Autodesk Inventor part; units mm, degrees
ref_plane "YZ Plane" through (0, 0, 0) normal (1, 0, 0) x (0, 1, 0)
ref_plane "XZ Plane" through (0, 0, 0) normal (0, 1, 0) x (-1, 0, 0)
ref_plane "XY Plane" through (0, 0, 0) normal (0, 0, 1) x (1, 0, 0)
sketch "Sketch1" plane through (0, 0, 0) normal (0, 0, 1) x (1, 0, 0)
  line L0 (0, 0) -> (30, 0)
  line L1 (30, 0) -> (30, 15)
  line L2 (30, 15) -> (0, 15)
  line L3 (0, 15) -> (0, 0)
  dimension "d0" = 30
  dimension "d1" = 15
extrude "Extrusion1" add sketch "Sketch1" along normal blind 25
sketch "Sketch2" plane through (0, 15, 0) normal (0, 1, 0) x (1, 0, 0)
  line L0 (30, 0) -> (0, 0)
  line L1 (0, 0) -> (0, -25)
  line L2 (30, -25) -> (0, -25)
  line L3 (30, 0) -> (30, -25)
  line L4 (7, -25) -> (23, -25)
  line L5 (23, -25) -> (23, -6)
  line L6 (23, -6) -> (7, -6)
  line L7 (7, -6) -> (7, -25)
  point P0 (0, 0)
  dimension "d5" = 16
  dimension "d27" = 7
  dimension "d28" = 6
extrude "Extrusion2" cut sketch "Sketch2" against normal up to next contours L2 L7 L6 L5
sketch "Sketch3" plane through (30, 0, 0) normal (1, 0, 0) x (0, 0, -1)
  circle A0 centre (-17.5, 7.5) radius 2.5
  line L0 (-25, 0) -> (-25, 15)
  line L1 (0, 15) -> (-25, 15)
  point P0 (0, 0)
  dimension "d10" = 5
  dimension "d11" = 7.5
  dimension "d12" = 7.5
extrude "Extrusion3" cut sketch "Sketch3" against normal through all
sketch "Sketch6" plane through (7, 15, 6) normal (0, 0, 1) x (1, 0, 0)
  circle A0 centre (8, -7.5) radius 5
  line L0 (0, 0) -> (16, 0)
  line L1 (16, 0) -> (16, -15)
  point P0 (-7, -15)
  dimension "d29" = 10
  dimension "d30" = 7.5
  dimension "d31" = 8
extrude "Extrusion6" cut sketch "Sketch6" against normal blind 4
sketch "Sketch7" plane through (15, 7.5, 2) normal (0, 0, 1) x (1, 0, 0)
  circle A0 centre (0, 0) radius 3.5
  point P0 (-15, -7.5)
  dimension "d34" = 7
extrude "Extrusion7" cut sketch "Sketch7" against normal up to next
properties part number "Arm_Pulley_Connector"
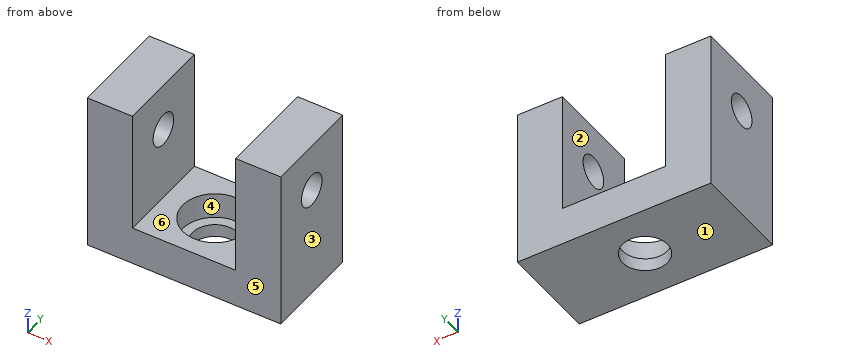
Geometry check sheet. Reference: the model listing, model coordinates, mm. Face numbers are marked on the shaded views. A direction names the side the tool comes from. Coordinates: 2 decimals unless noted, no trailing zeros. Order: outer loops, then holes, each group sorted by start corner. A loop starts at its lowest first (then second) coordinate and runs counter-clockwise, first axis right, second up. Notation, with made-up numbers: M 38,-19 L 84,-19 A26 ccw 84,6 Z; hole C 44,37.5 d1. An arc over 180 degrees is marked long. Use CSV: the item, a comma, the result in double quotes.
Item 1: Gauge pin test, flat ends, axial feed: pin 1 Ø3 at (x, y) = (14, 6.5) entering from +Z; pin 2 Ø5 at (x, y) = (19, 3.5) entering from +Z; pin 3 Ø8 at (y, z) = (7.5, 17.5) entering from -X. Record the tip position at first contact, or that the pin passes through.
Returned:
pin 1,"passes through"
pin 2,"stops at z = 6"
pin 3,"stops at x = 0"
Item 2: Cross-section at A-A on y = 7.5. Record the cut outline in (x, z).
Returned:
outline,"M 0,0 L 11.5,0 L 11.5,2 L 10,2 L 10,6 L 7,6 L 7,15 L 0,15 Z; M 0,20 L 7,20 L 7,25 L 0,25 Z; M 18.5,0 L 30,0 L 30,15 L 23,15 L 23,6 L 20,6 L 20,2 L 18.5,2 Z; M 23,20 L 30,20 L 30,25 L 23,25 Z"
Item 3: Thickness scan on line 1 along X through (y, z) = (6, 24.25); line 2 along Y through (x, z) = (15, 1.5); line 3 along Y through (x, z) = (15, 4.3). Record the ranges inside material, lowest first.
Returned:
line 1,"x = 0 to 7, 23 to 30"
line 2,"y = 0 to 4, 11 to 15"
line 3,"y = 0 to 2.5, 12.5 to 15"
Item 4: Cross-section at D-D on z = 17.5. Record the cut outline in (x, y).
Returned:
outline,"M 0,0 L 7,0 L 7,5 L 0,5 Z; M 0,10 L 7,10 L 7,15 L 0,15 Z; M 23,0 L 30,0 L 30,5 L 23,5 Z; M 23,10 L 30,10 L 30,15 L 23,15 Z"
Item 5: Cross-section at B-B on z = 13. Record the cut outline in (x, y).
Returned:
outline,"M 0,0 L 7,0 L 7,15 L 0,15 Z; M 23,0 L 30,0 L 30,15 L 23,15 Z"
Item 6: Cross-section at C-C on x = 15. Record the cut outline in (y, z).
Returned:
outline,"M 0,0 L 4,0 L 4,2 L 2.5,2 L 2.5,6 L 0,6 Z; M 11,0 L 15,0 L 15,6 L 12.5,6 L 12.5,2 L 11,2 Z"
Item 7: Mould release check, pull along X, two halves, no side actions. Record for the marked faces 3, 4, 5 and 6: pulls with the +X half, pulls with the -X half, needs draft (parallel to the pull), parting line crosses it, or undercut.
Returned:
face 3,"pulls with the +X half"
face 4,"undercut"
face 5,"needs draft"
face 6,"undercut"
Item 8: Tool access check on the marked faces 1 and 2. Record the directions out of +Z, -Z, +X, -X, +Y, -Y that give a thin tool (end or side, any length) a straight path to the whole face; none if there is none.
Returned:
face 1,"-Z, +X, -X, +Y, -Y"
face 2,"+Z, +Y, -Y"
